Here's the drawing with two shaded views (mm, measured from the low corner). I have some questions. A direction names the side the tool comes from. Give positions to 0.01 mm unless a question says otherwise; leave off trailing zeros. Write each loop counter-clockwise with the first axis right and the second up, starting at its lowest first coordinate (ties: lowest second). Pieces come first, ordered by that corner, then holes. Notation, with made-up numbers: M 43.5,0.5 L 79.5,0.5 A20 ccw 79.5,25.5 Z; hole C 63,28 d1. An arc over 180 degrees is marked long. Answer as CSV lines item,"result". Start each with the question number.
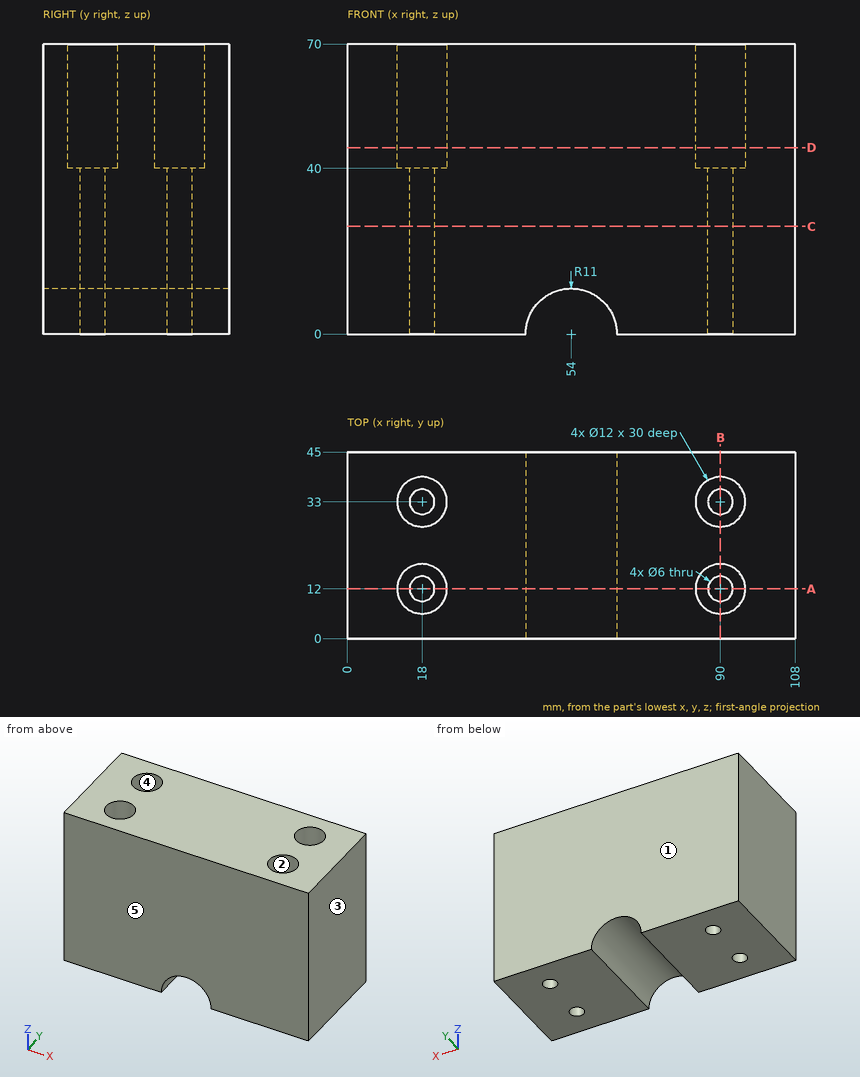
1. Imagine slicing it at B-B, the plane x = 90. Please give me the cut outline in (y, z).
2. Please list where these lines run through material, in increasing order: line 1 (Y direction, x = 90, z = 48.25); line 2 (Y direction, x = 18, z = 25.5); line 3 (X direction, y = 34, z = 49).
3. Thinking about a two-plate mould opening in X: for the marked faces 3, 4 and 5, which applies, pulls with the +X half, pulls with the -X half, needs draft (parallel to the pull), parting line crosses it, or undercut?
4. On a 3-axis mill with a long thin cutter (end or side, diameter ignored), from which of +Z, -Z, +X, -X, +Y, -Y can I reach the whole of each face in a straight line? I mean the marked faces 1 and 2. Say none if no direction works.
5. Imagine slicing it at C-C, the plane z = 26. Please give me the cut outline in (x, y).
6. Imagine slicing it at D-D, the plane z = 45. Please give me the cut outline in (x, y), plus the area to 3 significant figures.
7. Will these pins go through, and if not, where does the flat tip stop? P1, Ø14, axis at x = 18, y = 33, coming from the +Z side; P2, Ø9.5, axis at x = 90, y = 12, coming from the +Z side; P3, Ø3.5, axis at x = 90, y = 33, coming from the -Z side; P4, Ø1, axis at x = 56, y = 27.5, coming from the -Z side.
8. Imagine slicing it at A-A, the plane y = 12. Please give me the cut outline in (x, z), plus the area to 3 significant figures.
Solutions:
1,outline,"M 0,0 L 9,0 L 9,40 L 6,40 L 6,70 L 0,70 Z; M 15,0 L 30,0 L 30,40 L 27,40 L 27,70 L 18,70 L 18,40 L 15,40 Z; M 36,0 L 45,0 L 45,70 L 39,70 L 39,40 L 36,40 Z"
2,line 1,"0 to 6, 18 to 27, 39 to 45"
2,line 2,"0 to 9, 15 to 30, 36 to 45"
2,line 3,"0 to 12.08, 23.92 to 84.08, 95.92 to 108"
3,face 3,"pulls with the +X half"
3,face 4,"undercut"
3,face 5,"needs draft"
4,face 1,"+Z, -Z, +X, -X, +Y"
4,face 2,"+Z"
5,outline,"M 0,0 L 108,0 L 108,45 L 0,45 Z; hole C 18,12 d6; hole C 18,33 d6; hole C 90,12 d6; hole C 90,33 d6"
6,outline,"M 0,0 L 108,0 L 108,45 L 0,45 Z; hole C 18,12 d12; hole C 18,33 d12; hole C 90,12 d12; hole C 90,33 d12"
6,area,"4,410 mm²"
7,P1,"z = 70"
7,P2,"z = 40"
7,P3,"through"
7,P4,"z = 10.71"
8,outline,"M 0,0 L 15,0 L 15,40 L 12,40 L 12,70 L 0,70 Z; M 21,0 L 43,0 A11 cw 65,0 L 87,0 L 87,40 L 84,40 L 84,70 L 24,70 L 24,40 L 21,40 Z; M 93,0 L 108,0 L 108,70 L 96,70 L 96,40 L 93,40 Z"
8,area,"6,170 mm²"
